Design review of the part built by this model. Coordinates are the model's own, in mm. Face numbers are marked on the shaded views. A direction names the side the tool comes from. Round coordinates to 2 decimals unless told otherwise and drop trailing zeros. Order: outer loops, then holes, each group sorted by start corner. A loop starts at its lowest first (then second) coordinate and runs counter-clockwise, first axis right, second up. Notation, with made-up numbers: (-38.75, 31) - (-30.75, 31) arc R18 cw to (-30.75, 49) - close; hole circle Ø1 at (47.5, -36). An arc over 180 degrees is marked (long way). Write item = value, one per line.
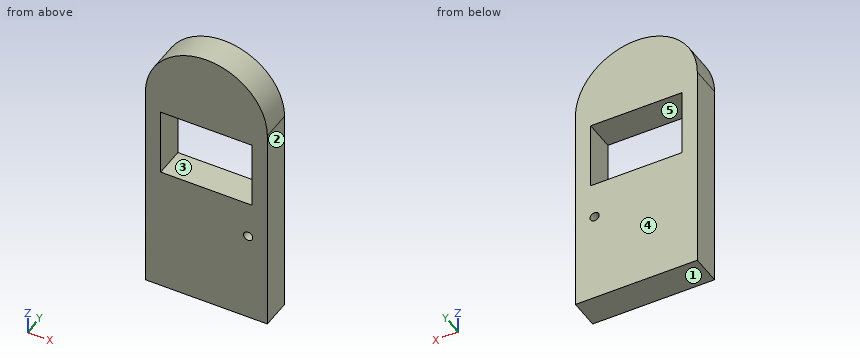
from build123d import *

# Parameters (mm, degrees)
F0_W     = 10.16
F0_H     = 17.78
F0_R     = 0.381
F1_DEPTH = 1.27


with BuildPart() as f1:
    # F0 (on Front) → F1 (new body, symmetric)
    with BuildSketch(Plane.XZ):
        with Locations((-5.08, 8.89)):
            Rectangle(F0_W, F0_H)
        with Locations((-1.60185, 7.633115)):
            Circle(F0_R, mode=Mode.SUBTRACT)
        Polygon((-8.89, 13.524802), (-8.89, 16.355868), (-5.08, 16.355868), (-1.27, 16.355868), (-1.27, 13.524802), (-1.27, 10.693735), (-5.08, 10.693735), (-8.89, 10.693735), align=None, mode=Mode.SUBTRACT)
        with BuildLine():
            Line((-10.16, 17.78), (0, 17.78))
            ThreePointArc((0, 17.78), (-5.08, 22.86), (-10.16, 17.78))
        make_face()
    extrude(amount=F1_DEPTH, both=True)


solid = f1.part
1) Clearance check with flat-ended pins moving along their axes: pin 1 Ø1.3 at (x, y) = (-7, 0) entering from +Z; pin 2 Ø1.5 at (y, z) = (-0.5, 19.5) entering from -X. State where each tip first meets the part, or that it passes through.
Findings:
pin_1 = 22.7
pin_2 = -10.07
2) We need section A-A on z = 13. Write out the cut boundary in (x, y), and give its area (3 significant figures).
Findings:
outline = (-10.16, -1.27) - (-8.89, -1.27) - (-8.89, 1.27) - (-10.16, 1.27) - close; (-1.27, -1.27) - (0, -1.27) - (0, 1.27) - (-1.27, 1.27) - close
area = 6.45 mm^2
3) We need section D-D on x = -1. Write out the cut boundary in (y, z).
Findings:
outline = (-1.27, 0) - (1.27, 0) - (1.27, 20.81) - (-1.27, 20.81) - close
4) For the marked faces 4 and 5, list the 3-axis set-ups (+Z, -Z, +X, -X, +Y, -Y) from which the entire face can be reached by the end or side of a thin tool; tool diameter is ignored.
Findings:
face_4 = +Z, -Z, +X, -X, +Y
face_5 = +Y, -Y
5) The part is to be moulded in two halves that separate along X. For the marked faces 1, 2 and 3, say which applies: released by +X, released by -X, zero draft, split by the parting line, or undercut.
Findings:
face_1 = zero draft
face_2 = released by +X
face_3 = undercut
6) We need section B-B on x = -5.08. Write out the cut boundary in (y, z).
Findings:
outline = (-1.27, 0) - (1.27, 0) - (1.27, 10.69) - (-1.27, 10.69) - close; (-1.27, 16.36) - (1.27, 16.36) - (1.27, 22.86) - (-1.27, 22.86) - close
7) To check wall thickness, follow L1, parallel to X at y = -0.4, z = 14.5; L2, parallel to Z at x = -8.75, y = 0.95; L3, parallel to Z at x = -7.5, y = -0.8. State the ranges of each line that lie inside material, in increasing order. Write a range as from..to.
Findings:
L1 = -10.16..-8.89, -1.27..0
L2 = 0..10.69, 16.36..21.29
L3 = 0..10.69, 16.36..22.25
8) We need section C-C on y = 0.05. Write out the cut boundary in (x, z).
Findings:
outline = (-10.16, 0) - (0, 0) - (0, 17.78) arc R5.08 ccw to (-10.16, 17.78) - close; hole (-8.89, 10.69) - (-1.27, 10.69) - (-1.27, 16.36) - (-8.89, 16.36) - close; hole circle Ø0.76 at (-1.6, 7.63)
